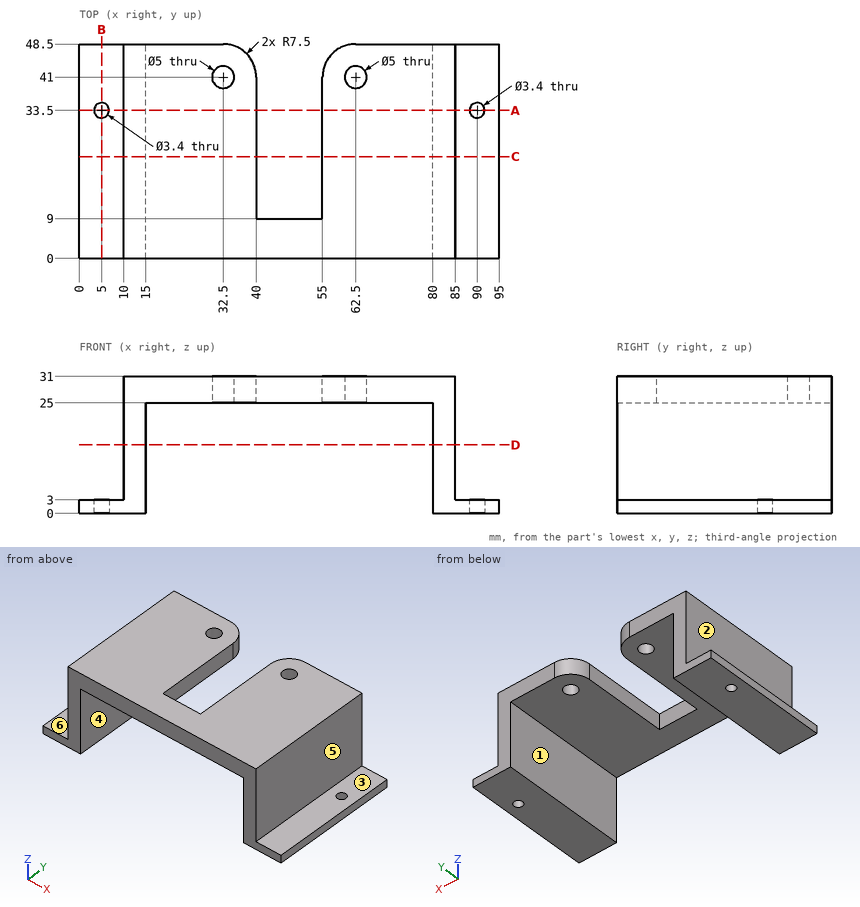
Could you check a few things on this drawing? It's one solid part, dimensions in mm from its lowest x, y, z. A direction names the side the tool comes from. Coordinates: 2 decimals unless noted, no trailing zeros. Write each loop counter-clockwise with the first axis right and the second up, starting at its lowest first coordinate (ties: lowest second). Pieces come first, ordered by that corner, then holes.
Q1. Imagine slicing it at B-B, the plane x = 5. List the corners of the cut face in (y, z) for me, plus the area to 3 significant figures.
Results found:
outline: (0, 0) - (31.8, 0) - (31.8, 3) - (0, 3) - close; (35.2, 0) - (48.5, 0) - (48.5, 3) - (35.2, 3) - close
area: 135 mm2
Q2. Please list where these lines run through material, in increasing order: L1, parallel to X at y = 11, z = 13.5; L2, parallel to X at y = 22.5, z = 26; L3, parallel to Y at x = 62.5, z = 26.75.
Results found:
L1: x = 10 to 15, 80 to 85
L2: x = 10 to 40, 55 to 85
L3: y = 0 to 38.5, 43.5 to 48.5
Q3. Which directions (+Z, -Z, +X, -X, +Y, -Y) give clear straight access to the entire face, cutting with the end or side of a thin tool? Please do the marked faces 4, 5 and 6.
Results found:
face 4: -Z, +Y, -Y
face 5: +Z, +X, +Y, -Y
face 6: +Z, -X, +Y, -Y
Q4. Imagine slicing it at A-A, the plane y = 33.5. List the corners of the cut face in (x, z) for me.
Results found:
outline: (0, 0) - (3.3, 0) - (3.3, 3) - (0, 3) - close; (6.7, 0) - (15, 0) - (15, 25) - (40, 25) - (40, 31) - (10, 31) - (10, 3) - (6.7, 3) - close; (55, 25) - (80, 25) - (80, 0) - (88.3, 0) - (88.3, 3) - (85, 3) - (85, 31) - (55, 31) - close; (91.7, 0) - (95, 0) - (95, 3) - (91.7, 3) - close
Q5. For P1, Ø1, axis at y = 33.5, z = 22, coming from the +X side; P2, Ø4, axis at y = 8, z = 15.5, coming from the -X side; P3, Ø6.5, axis at x = 44.5, z = 28.5, coming from the +Y side, each with a flat end and sliding along its axis, tell me the tip position at first contact or that it passes through.
Results found:
P1: stops at x = 85
P2: stops at x = 10
P3: stops at y = 9
Q6. If we mould it in two halves opening along X, with no side actions, what happens to the marked faces 1, 2 and 3? For each: +X half, -X half, draft (parallel to the pull), parting line (faces both ways), or undercut.
Results found:
face 1: undercut
face 2: -X half
face 3: draft
Q7. Imagine slicing it at C-C, the plane y = 23. List the corners of the cut face in (x, z) for me, plus the area to 3 significant figures.
Results found:
outline: (0, 0) - (15, 0) - (15, 25) - (40, 25) - (40, 31) - (10, 31) - (10, 3) - (0, 3) - close; (55, 25) - (80, 25) - (80, 0) - (95, 0) - (95, 3) - (85, 3) - (85, 31) - (55, 31) - close
area: 670 mm2
Q8. Imagine slicing it at D-D, the plane z = 15.5. List the corners of the cut face in (x, y) for me.
Results found:
outline: (10, 0) - (15, 0) - (15, 48.5) - (10, 48.5) - close; (80, 0) - (85, 0) - (85, 48.5) - (80, 48.5) - close
